Autodesk Inventor part; units mm, degrees
ref_plane "YZ Plane" through (0, 0, 0) normal (1, 0, 0) x (0, 1, 0)
ref_plane "XZ Plane" through (0, 0, 0) normal (0, 1, 0) x (-1, 0, 0)
ref_plane "XY Plane" through (0, 0, 0) normal (0, 0, 1) x (1, 0, 0)
sketch "Sketch1" plane through (0, 0, 0) normal (0, 0, 1) x (1, 0, 0)
  circle A0 centre (0, 0) radius 6.35
  dimension "d0" = 12.7
extrude "Extrusion1" add sketch "Sketch1" along normal mid plane 184.15
sketch "Sketch2" plane through (0, 0, 92.075) normal (0, 0, 1) x (1, 0, 0)
  circle A0 centre (0, 0) radius 6.35
hole "Hole1" at (0, 0, 92.075) direction (0, 0, -1) diameter 4.9784 depth 19.05 tip angle 118
mirror "Mirror1" about plane through (0, 0, 0) normal (0, 0, 1) of "Hole1"
properties part number "wheel_shaft" material "Steel"
Can you work these out from the model? Positions are in its coordinate system, mm. A direction names the side the tool comes from. Coordinates: 2 decimals unless noted, no trailing zeros. Write each loop counter-clockwise with the first axis right and the second up, starting at its lowest first coordinate (ties: lowest second). Pieces come first, ordered by that corner, then holes. Notation, with made-up numbers: M 22.5,7.25 L 56.5,7.25 A20 ccw 56.5,18.25 Z; hole C 89.5,68.25 d4. An arc over 180 degrees is marked long. Answer as CSV lines item,"result".
Item 1: We'd pull the mould along Y, two halves only. Please class faces 1 (the cylindrical face through (-1.38, 6.2, -1.29)), 2 (the flat face through (3, 0, -92.075)), 3 (the conical face through (-0.422, 0.094, 71.789)), 4 (the cylindrical face through (0.748, -2.374, -82.417)): +Y half, -Y half, draft (parallel to the pull), parting line (faces both ways), or undercut.
Geometry results:
face 1,"parting line"
face 2,"draft"
face 3,"undercut"
face 4,"undercut"
Item 2: I'm going to push flat-ended pins straight in: P1, Ø4.5, axis at x = 0, y = 0, coming from the +Z side; P2, Ø4, axis at y = 4, z = 54.5, coming from the -X side; P3, Ø3, axis at y = 4.5, z = -29.5, coming from the -X side. Where does each tip first touch, or does it pass through?
Geometry results:
P1,"stops at z = 72.88"
P2,"stops at x = -6.03"
P3,"stops at x = -5.6"
Item 3: Please list where these lines run through material, in increasing order: line 1 along Y through (x, z) = (0, 86.5); line 2 along X through (y, z) = (0.25, -57); line 3 along Y through (x, z) = (-0.75, -80.5).
Geometry results:
line 1,"y = -6.35 to -2.49, 2.49 to 6.35"
line 2,"x = -6.35 to 6.35"
line 3,"y = -6.31 to -2.37, 2.37 to 6.31"
Item 4: Imagine slicing it at A-A on z = -7. List the corners of the cut face in (x, y) for me.
Geometry results:
outline,"C 0,0 d12.7"
Item 5: Imagine slicing it at B-B on y = -4.5. List the corners of the cut face in (x, z) for me (3 decimals).
Geometry results:
outline,"M -4.48,-92.075 L 4.48,-92.075 L 4.48,92.075 L -4.48,92.075 Z"
Item 6: On a 3-axis mill with a long thin cutter (end or side, diameter ignored), from which of +Z, -Z, +X, -X, +Y, -Y can I reach the whole of each face in a straight line? I mean faces 5 (the cylindrical face through (-0.748, -2.374, 82.417)), 6 (the flat face through (3, 0, 92.075)). Say none if no direction works.
Geometry results:
face 5,"+Z"
face 6,"+Z, +X, -X, +Y, -Y"
